Part model, mm, in its own coordinate system. Face numbers are marked on the shaded views. A direction names the side the tool comes from. Coordinates: 2 decimals unless noted, no trailing zeros. Loops run counter-clockwise (first coordinate to the right, second up) from the corner with the lowest first, then second, coordinate; pieces in that order, holes last. Notation, with made-up numbers: (28.25, 32) -> (86.25, 32) arc R23 ccw to (86.25, 50) -> close; hole circle Ø6 at (58.5, 60.5). An arc over 180 degrees is marked (long way). One line per question, with ' | ' between items. Start each with the question number.
1) 3-axis set-ups, long thin cutter, end or side, ignore diameter. For the marked faces 4, 5 and 6: which of +Z, -Z, +X, -X, +Y, -Y reach the whole face in a straight line?
2) Cut at D-D (x = 24.3). List the corners of the cut face in (y, z).
3) Drop flat-ended pins along their axis: pin 1 (3.5 mm diameter, centred on y = -2.5, z = -11, fed in from +X); pin 2 (17.5 mm diameter, centred on x = 13.5, z = -27.5, fed in from -Y); pin 3 (2.5 mm diameter, centred on x = -24.3, z = -33.55, fed in from +Y); pin 4 (10 mm diameter, centred on x = 2, z = -3, fed in from +Y). Give the stop position or say it passes through.
4) Cut at A-A (y = -4.9). List the corners of the cut face in (x, z), plus the area to 3 significant figures.
5) Cut at B-B (y = -9). List the corners of the cut face in (x, z), plus the area to 3 significant figures.
6) Two-plate mould, pull along Z, no slides. Class the marked faces 1, 2 and 3: released by +Z, released by -Z, zero draft, split by the parting line, or undercut.
7) Probe L1, parallel to X at y = 10.8, z = -33.55; L2, parallel to Y at x = 24.3, z = -12; L3, parallel to Z at x = 13, y = -8.5. List the from-to ranges inside material, lowest first. Write a range as from..to.
8) Cut at C-C (z = -23.55). List the corners of the cut face in (x, y).
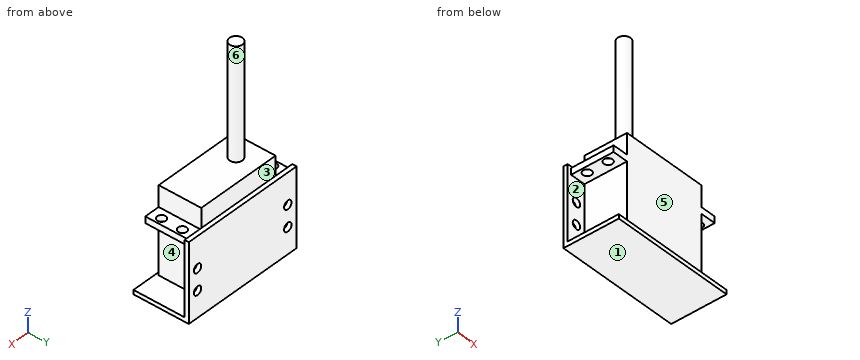
from build123d import *

# Parameters (mm, degrees)
SKETCH2_W           = 40
SKETCH2_H           = 20
SKETCH2_R           = 7
SKETCH2_R_2         = 3
BOSS_EXTRUDE1_DEPTH = 40.45
BOSS_EXTRUDE2_START = -12.8
SKETCH2_3_W         = 7.22
SKETCH2_3_H         = 20
SKETCH2_3_R         = 2
BOSS_EXTRUDE2_DEPTH = 3
SKETCH2_4_R         = 3
BOSS_EXTRUDE3_DEPTH = 52
SKETCH3_W           = 58
SKETCH3_H           = 36.7
SKETCH3_R           = 2
BOSS_EXTRUDE4_DEPTH = 2
SKETCH4_W           = 58
SKETCH4_H           = 2
BOSS_EXTRUDE5_DEPTH = 24


with BuildPart() as part:
    # Sketch2 → Boss-Extrude1 (new body)
    # profile 1 of 3: a face of its own
    with BuildSketch(Plane.XY):
        Rectangle(SKETCH2_W, SKETCH2_H)
        with Locations((-10.15, 0)):
            Circle(SKETCH2_R, mode=Mode.SUBTRACT)
    # profile 2 of 3: a face of its own
    with BuildSketch(Plane.XY):
        with Locations((-10.15, 0)):
            Circle(SKETCH2_R)
    # profile 3 of 3: a face of its own
    with BuildSketch(Plane.XY):
        with Locations((-10.15, 0)):
            Circle(SKETCH2_R_2)
    extrude(amount=-BOSS_EXTRUDE1_DEPTH)

    # Sketch2_3 → Boss-Extrude2 (add)
    # profile 1 of 2: a face of its own
    with BuildSketch(Plane.XY.offset(BOSS_EXTRUDE2_START)):
        with Locations((-23.61, 0)):
            Rectangle(SKETCH2_3_W, SKETCH2_3_H)
        with Locations((-24.3, -4.9)):
            Circle(SKETCH2_3_R, mode=Mode.SUBTRACT)
        with Locations((-24.3, 4.9)):
            Circle(SKETCH2_3_R, mode=Mode.SUBTRACT)
    # profile 2 of 2: a face of its own
    with BuildSketch(Plane.XY.offset(BOSS_EXTRUDE2_START)):
        with Locations((23.61, 0)):
            Rectangle(SKETCH2_3_W, SKETCH2_3_H)
        with Locations((24.3, -4.9)):
            Circle(SKETCH2_3_R, mode=Mode.SUBTRACT)
        with Locations((24.3, 4.9)):
            Circle(SKETCH2_3_R, mode=Mode.SUBTRACT)
    extrude(amount=BOSS_EXTRUDE2_DEPTH)

    # Sketch2_4 → Boss-Extrude3 (add)
    with BuildSketch(Plane.XY):
        with Locations(Location((-10.15, 0, 0), (0, 0, 180))):
            Circle(SKETCH2_4_R)
    extrude(amount=BOSS_EXTRUDE3_DEPTH)

    # Sketch3 → Boss-Extrude4 (add)
    with BuildSketch(Plane(origin=(0, 10, 0), x_dir=(1, 0, 0), z_dir=(0, 1, 0))):
        with Locations((0, 27.4)):
            Rectangle(SKETCH3_W, SKETCH3_H)
        with Locations(Location((-24.3, 33.55, 0), (0, 0, 270))):
            Circle(SKETCH3_R, mode=Mode.SUBTRACT)
        with Locations(Location((-24.3, 23.55, 0), (0, 0, 270))):
            Circle(SKETCH3_R, mode=Mode.SUBTRACT)
        with Locations(Location((24.3, 33.55, 0), (0, 0, 270))):
            Circle(SKETCH3_R, mode=Mode.SUBTRACT)
        with Locations(Location((24.3, 23.55, 0), (0, 0, 270))):
            Circle(SKETCH3_R, mode=Mode.SUBTRACT)
    extrude(amount=BOSS_EXTRUDE4_DEPTH)

    # Sketch4 → Boss-Extrude5 (add)
    with BuildSketch(Plane.XZ.offset(-10)):
        with Locations((0, -44.75)):
            Rectangle(SKETCH4_W, SKETCH4_H)
    extrude(amount=BOSS_EXTRUDE5_DEPTH)


solid = part.part
Reported:
1) face 4: +X, -Y | face 5: +Z, +X, -X, -Y | face 6: +Z
2) outline: (-14, -45.75) -> (12, -45.75) -> (12, -35.55) -> (10, -35.55) -> (10, -43.75) -> (-14, -43.75) -> close; (-10, -12.8) -> (-6.9, -12.8) -> (-6.9, -9.8) -> (-10, -9.8) -> close; (-2.9, -12.8) -> (2.9, -12.8) -> (2.9, -9.8) -> (-2.9, -9.8) -> close; (6.9, -12.8) -> (10, -12.8) -> (10, -21.55) -> (12, -21.55) -> (12, -9.05) -> (10, -9.05) -> (10, -9.8) -> (6.9, -9.8) -> close; (10, -31.55) -> (12, -31.55) -> (12, -25.55) -> (10, -25.55) -> close
3) pin 1: stops at x = 27.22 | pin 2: stops at y = -10 | pin 3: passes through | pin 4: stops at y = 10
4) outline: (-29, -45.75) -> (29, -45.75) -> (29, -43.75) -> (-29, -43.75) -> close; (-27.22, -12.8) -> (-26.3, -12.8) -> (-26.3, -9.8) -> (-27.22, -9.8) -> close; (-22.3, -12.8) -> (-20, -12.8) -> (-20, -40.45) -> (20, -40.45) -> (20, -12.8) -> (22.3, -12.8) -> (22.3, -9.8) -> (20, -9.8) -> (20, 0) -> (-20, 0) -> (-20, -9.8) -> (-22.3, -9.8) -> close; (26.3, -12.8) -> (27.22, -12.8) -> (27.22, -9.8) -> (26.3, -9.8) -> close | area: 1,750 mm²
5) outline: (-29, -45.75) -> (29, -45.75) -> (29, -43.75) -> (-29, -43.75) -> close; (-27.22, -12.8) -> (-20, -12.8) -> (-20, -40.45) -> (20, -40.45) -> (20, -12.8) -> (27.22, -12.8) -> (27.22, -9.8) -> (20, -9.8) -> (20, 0) -> (-20, 0) -> (-20, -9.8) -> (-27.22, -9.8) -> close | area: 1,780 mm²
6) face 1: released by -Z | face 2: undercut | face 3: zero draft
7) L1: x = -29..-26.3, -22.3..22.3, 26.3..29 | L2: y = -10..-6.9, -2.9..2.9, 6.9..12 | L3: z = -45.75..-43.75, -40.45..0
8) outline: (-29, 10) -> (-26.3, 10) -> (-26.3, 12) -> (-29, 12) -> close; (-22.3, 10) -> (-20, 10) -> (-20, -10) -> (20, -10) -> (20, 10) -> (22.3, 10) -> (22.3, 12) -> (-22.3, 12) -> close; (26.3, 10) -> (29, 10) -> (29, 12) -> (26.3, 12) -> close
